from build123d import *
from build123d.topology import SkipClean

# Parameters (mm, degrees)
SKETCH2_W           = 70
SKETCH2_H           = 17
BOSS_EXTRUDE1_DEPTH = 2
SKETCH3_W           = 35
SKETCH3_H           = 17
BOSS_EXTRUDE2_DEPTH = 15.7
SKETCH4_W           = 23
SKETCH4_H           = 12.5
CUT_EXTRUDE1_DEPTH  = 41.131533736
SKETCH6_R           = 0.8
CUT_EXTRUDE2_DEPTH  = 8
CUT_EXTRUDE3_DEPTH  = 8
SKETCH9_W           = 18
SKETCH9_H           = 2
BOSS_EXTRUDE3_DEPTH = 18
FILLET1_R           = 8
FILLET2_R           = 8
FILLET3_START       = -8.5
FILLET3_DEPTH       = 17
FILLET3_START_2     = -25.5
FILLET3_2_DEPTH     = 8
SKETCH11_R          = 1.5
CUT_EXTRUDE4_DEPTH  = 18


with BuildPart() as part:
    # Sketch2 → Boss-Extrude1 (new body)
    with BuildSketch(Plane(origin=(0, 0, 0), x_dir=(1, 0, 0), z_dir=(0, 1, 0))):
        Rectangle(SKETCH2_W, SKETCH2_H)
    extrude(amount=BOSS_EXTRUDE1_DEPTH)

    # Sketch3 → Boss-Extrude2 (add)
    with BuildSketch(Plane(origin=(0, 2, 0), x_dir=(1, 0, 0), z_dir=(0, 1, 0))):
        Rectangle(SKETCH3_W, SKETCH3_H)
    extrude(amount=BOSS_EXTRUDE2_DEPTH)

    # Sketch4 → Cut-Extrude1 (cut, through all)
    with BuildSketch(Plane(origin=(0, 17.7, 0), x_dir=(1, 0, 0), z_dir=(0, 1, 0))):
        Rectangle(SKETCH4_W, SKETCH4_H)
    extrude(amount=-CUT_EXTRUDE1_DEPTH, mode=Mode.SUBTRACT)

    # Sketch6 → Cut-Extrude2 (cut)
    with BuildSketch(Plane(origin=(0, 17.7, 0), x_dir=(1, 0, 0), z_dir=(0, 1, 0))):
        with Locations(Location((13.65, 0, 0), (0, 0, 270))):
            Circle(SKETCH6_R)
        with Locations(Location((-13.65, 0, 0), (0, 0, 90))):
            Circle(SKETCH6_R)
    extrude(amount=-CUT_EXTRUDE2_DEPTH, mode=Mode.SUBTRACT)

    # Sketch7 → Cut-Extrude3 (cut)
    with BuildSketch(Plane.ZY.offset(17.5)):
        with BuildLine():
            Line((-4.5, 5.8), (-4.5, 3.8))
            Line((-4.5, 3.8), (4.5, 3.8))
            Line((4.5, 3.8), (4.5, 5.8))
            ThreePointArc((4.5, 5.8), (0, 10.3), (-4.5, 5.8))
        make_face()
    extrude(amount=-CUT_EXTRUDE3_DEPTH, mode=Mode.SUBTRACT)

    # Sketch9 → Boss-Extrude3 (add)
    with BuildSketch(Plane.XY.offset(8.5)):
        with Locations((0, 1)):
            Rectangle(SKETCH9_W, SKETCH9_H)
    boss_extrude3 = extrude(amount=BOSS_EXTRUDE3_DEPTH)

    # Mirror1: Boss-Extrude3 across plane
    add(boss_extrude3.mirror(Plane.XY))

    # Fillet1
    fillet1_edges = [part.edges().sort_by_distance(p)[0] for p in [
        (0, 2, 8.5),
    ]]
    fillet(fillet1_edges, radius=FILLET1_R)

    # Fillet2
    fillet2_edges = [part.edges().sort_by_distance(p)[0] for p in [
        (-9, 1, -8.5),
        (-9, 5, 8.5),
        (9, 5, 8.5),
        (9, 1, -8.5),
        (0, 2, -8.5),
        (17.5, 2, 0),
    ]]
    fillet(fillet2_edges, radius=FILLET2_R)

    # Fillet3: read off the stored shape, not the designer's step
    # Fillet3 outline → Fillet3 (add)
    with BuildSketch(Plane.XY.offset(FILLET3_START)):
        with BuildLine():
            ThreePointArc((-17.5, 10.00000495), (-19.843144, 4.343147501), (-25.5, 2))
            Line((-25.5, 2), (-17.5, 2))
            Line((-17.5, 2), (-17.5, 10.00000495))
        make_face()
    extrude(amount=FILLET3_DEPTH)

    # Fillet3 2 outline → Fillet3 2 (cut)
    with SkipClean():  # the faces are left unmerged after this step: merging them gives an invalid solid
        with BuildSketch(Plane.YZ.offset(FILLET3_START_2)):
            with BuildLine():
                ThreePointArc((5.799996271, -4.5), (10.3, -1.865e-06), (5.8, 4.5))
                Line((5.8, 4.5), (3.8, 4.5))
                Line((3.8, 4.5), (3.8, -4.5))
                Line((3.8, -4.5), (5.799996271, -4.5))
            make_face()
        extrude(amount=FILLET3_2_DEPTH, mode=Mode.SUBTRACT)

    # Sketch11 → Cut-Extrude4 (cut)
    with SkipClean():  # the faces are left unmerged after this step: merging them gives an invalid solid
        with BuildSketch(Plane(origin=(0, 2, 0), x_dir=(1, 0, 0), z_dir=(0, 1, 0))):
            with Locations(Location((4.772736854, 21.529356347, 0), (0, 0, 270))):
                Circle(SKETCH11_R)
            with Locations(Location((-4.821076753, 21.529356347, 0), (0, 0, 270))):
                Circle(SKETCH11_R)
            with Locations(Location((4.772736854, -22.011031546, 0), (0, 0, 270))):
                Circle(SKETCH11_R)
            with Locations(Location((-4.821076753, -22.011031546, 0), (0, 0, 270))):
                Circle(SKETCH11_R)
            with Locations(Location((30.348655276, 4.696340636, 0), (0, 0, 270))):
                Circle(SKETCH11_R)
            with Locations(Location((30.348655276, -4.691151825, 0), (0, 0, 270))):
                Circle(SKETCH11_R)
            with Locations(Location((-30.467199024, -4.691151825, 0), (0, 0, 270))):
                Circle(SKETCH11_R)
            with Locations(Location((-30.467199024, 4.696340636, 0), (0, 0, 270))):
                Circle(SKETCH11_R)
        extrude(amount=-CUT_EXTRUDE4_DEPTH, mode=Mode.SUBTRACT)


solid = part.part
Could you check a few things on this model? Use its own coordinates, in mm. A direction names the side the tool comes from. Round coordinates to 2 decimals unless told otherwise and drop trailing zeros. Write each loop counter-clockwise with the first axis right and the second up, starting at its lowest first coordinate (ties: lowest second). Pieces come first, ordered by that corner, then holes. Notation, with made-up numbers: (27, -7.5) - (76, -7.5) arc R32 ccw to (76, 30.5) - close; hole circle Ø8 at (25, -33.75). An arc over 180 degrees is marked (long way). Put each result on its own line as item: value. Start each with the question number.
(1) I want a section at B-B, the plane x = -10.5. Please give me the cut outline in (y, z), plus the area to 3 significant figures.
(2) I want a section at A-A, the plane z = 0. Please give me the cut outline in (x, y).
(3) Will these pins go through, and if not, where does the flat tip stop? pin 1 (5 mm diameter, centred on x = -6, z = -12.5, fed in from +Y); pin 2 (8 mm diameter, centred on x = 2.5, z = -24, fed in from +Y); pin 3 (5.5 mm diameter, centred on x = 12.5, y = 12, fed in from -Z).
(4) I need wall thicknesses on probe 1 along X at (y, z) = (16.25, 0); probe 2 along X at (y, z) = (15.75, 3.5); probe 3 along Y at (x, z) = (-4.5, -18). Which ranges of each line are inside material? Lowest first, please.
(5) I want a section at D-D, the plane x = -22. Please give me the cut outline in (y, z).
(6) Thinking about a two-plate mould opening in X: for faces 1 (the flat face through (-4, 17.7, 7)), 2 (the flat face through (-17.5, 14, 0)), 3 (the flat face through (0, 9, -6.25)), which applies, released by +X, released by -X, zero draft, split by the parting line, or undercut?
(7) I want a section at C-C, the plane z = 14.5. Please give me the cut outline in (x, y).
(8) For faces 4 (the flat face through (-9, 1, 21)), 5 (the flat face through (0, 2, 21)), 6 (the flat face through (9, 1, -21)), 7 (the cylindrical face through (14.443, 13.756, -0.104)), which set-ups out of +Z, -Z, +X, -X, +Y, -Y let a thin tool reach every point of the face, with its end or its side?
Here are the results:
1. outline: (0, -11.84) - (3.5, -11.84) arc R8 cw to (10, -8.5) - (17.7, -8.5) - (17.7, -6.25) - (0, -6.25) - close; (0, 6.25) - (17.7, 6.25) - (17.7, 8.5) - (10, 8.5) arc R8 cw to (3.5, 11.84) - (0, 11.84) - close
1. area: 116 mm^2
2. outline: (-35, 0) - (-11.5, 0) - (-11.5, 3.8) - (-20.44, 3.8) arc R8 cw to (-25.5, 2) - (-35, 2) - close; (-17.5, 10.3) - (-14.45, 10.3) - (-14.45, 17.7) - (-17.5, 17.7) - close; (-12.85, 10.3) - (-11.5, 10.3) - (-11.5, 17.7) - (-12.85, 17.7) - close; (11.5, 0) - (35, 0) - (35, 2) - (25.5, 2) arc R8 cw to (17.5, 10) - (17.5, 17.7) - (14.45, 17.7) - (14.45, 9.7) - (12.85, 9.7) - (12.85, 17.7) - (11.5, 17.7) - close
3. pin 1: stops at y = 5.34
3. pin 2: stops at y = 2
3. pin 3: stops at z = -8.54
4. probe 1: x = -17.5 to -14.45, -12.85 to -11.5, 11.5 to 12.85, 14.45 to 17.5
4. probe 2: x = -17.5 to -11.5, 11.5 to 17.5
4. probe 3: y = 0 to 2
5. outline: (0, -8.5) - (2.81, -8.5) - (2.81, 8.5) - (0, 8.5) - close
6. face 1: zero draft
6. face 2: released by -X
6. face 3: undercut
7. outline: (-9.25, 0) - (9.25, 0) - (9.25, 2.25) - (-9.25, 2.25) - close
8. face 4: +Z, -X, +Y, -Y
8. face 5: +Z, +X, -X, +Y
8. face 6: -Z, +X, +Y, -Y
8. face 7: +Y
